Could you check a few things on this model? Use its own coordinates, in mm. Coordinates: 2 decimals unless noted, no trailing zeros. Loops run counter-clockwise (first coordinate to the right, second up) from the corner with the lowest first, then second, coordinate; pieces in that order, holes last. Notation, with made-up numbers: (2, 46) - (47, 46) arc R31 cw to (47, 73) - close; hole circle Ø7 at (28.5, 36.5). An arc over 180 degrees is marked (long way). One line per item, written item: value. Start each with the question number.
(1) If we section it at C-C on y = 0.6: Count the separate pieces of the cut face and the enclosed holes in it, then the cut area to 3 significant figures.
(2) If we section it at B-B on z = 1.5: Write out the boundary of the cut face in (x, y), then the cut area to 3 significant figures.
(3) If we section it at A-A on x = 10: Write out the boundary of the cut face in (y, z).
(4) If I drill on line 1 along X through (y, z) = (3, -9); line 2 along Z through (x, y) = (53, 3.05) (3 decimals); line 3 along Z through (x, y) = (-32, 1), over which ranges is the centre line in solid material (lowest first)? Write a range as from..to.
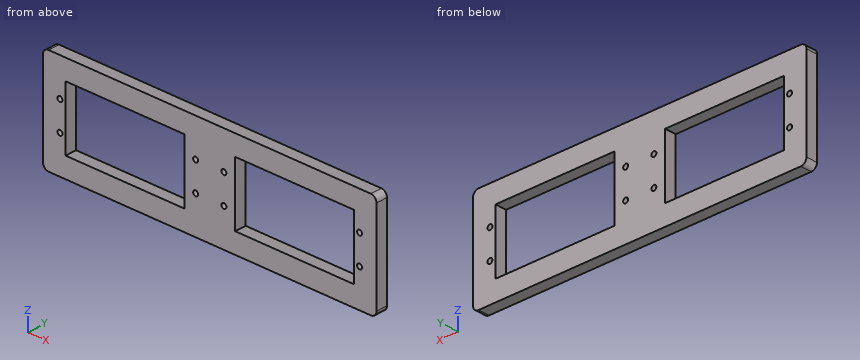
```python
from build123d import *

# Parameters (mm, degrees)
SKETCH2_W           = 42
SKETCH2_H           = 22
BOSS_EXTRUDE1_DEPTH = 4
SKETCH3_R           = 0.875
CUT_EXTRUDE1_DEPTH  = 10
SKETCH4_R           = 0.875
CUT_EXTRUDE2_DEPTH  = 10


with BuildPart() as part:
    # Sketch2 → Boss-Extrude1 (new body)
    with BuildSketch(Plane(origin=(0, 0, 0), x_dir=(1, 0, 0), z_dir=(0, 1, 0))):
        with BuildLine():
            Line((-57, 18), (57, 18))
            ThreePointArc((57, 18), (58.414213562, 17.414213562), (59, 16))
            Line((59, 16), (59, -16))
            ThreePointArc((59, -16), (58.414213562, -17.414213562), (57, -18))
            Line((57, -18), (-57, -18))
            ThreePointArc((-57, -18), (-58.414213562, -17.414213562), (-59, -16))
            Line((-59, -16), (-59, 16))
            ThreePointArc((-59, 16), (-58.414213562, 17.414213562), (-57, 18))
        make_face()
        with Locations((-30, 0)):
            Rectangle(SKETCH2_W, SKETCH2_H, mode=Mode.SUBTRACT)
        with Locations((30, 0)):
            Rectangle(SKETCH2_W, SKETCH2_H, mode=Mode.SUBTRACT)
    extrude(amount=BOSS_EXTRUDE1_DEPTH)

    # Sketch3 → Cut-Extrude1 (cut)
    with BuildSketch(Plane.XZ):
        with Locations(Location((-53, 5, 0), (0, 0, 270))):
            Circle(SKETCH3_R)
        with Locations(Location((-53, -5, 0), (0, 0, 270))):
            Circle(SKETCH3_R)
    cut_extrude1 = extrude(amount=-CUT_EXTRUDE1_DEPTH, mode=Mode.SUBTRACT)

    # Sketch4 → Cut-Extrude2 (cut)
    with BuildSketch(Plane.XZ):
        with Locations(Location((-5, 5, 0), (0, 0, 270))):
            Circle(SKETCH4_R)
        with Locations(Location((-5, -5, 0), (0, 0, 270))):
            Circle(SKETCH4_R)
    cut_extrude2 = extrude(amount=-CUT_EXTRUDE2_DEPTH, mode=Mode.SUBTRACT)

    # Mirror1: Cut-Extrude1, Cut-Extrude2 across plane
    add(cut_extrude1.mirror(Plane(origin=(0, 0, 0), x_dir=(0, 0, 1), z_dir=(1, 0, 0))), mode=Mode.SUBTRACT)
    add(cut_extrude2.mirror(Plane(origin=(0, 0, 0), x_dir=(0, 0, 1), z_dir=(1, 0, 0))), mode=Mode.SUBTRACT)


solid = part.part
```
Values:
1. separate pieces: 1
1. enclosed holes: 10
1. area: 2,380 mm2
2. outline: (-59, 0) - (-51, 0) - (-51, 4) - (-59, 4) - close; (-9, 0) - (9, 0) - (9, 4) - (-9, 4) - close; (51, 0) - (59, 0) - (59, 4) - (51, 4) - close
2. area: 136 mm2
3. outline: (0, -18) - (4, -18) - (4, -11) - (0, -11) - close; (0, 11) - (4, 11) - (4, 18) - (0, 18) - close
4. line 1: x = -59..-51, -9..9, 51..59
4. line 2: z = -18..-5.875, -4.125..4.125, 5.875..18
4. line 3: z = -18..-11, 11..18
